Check sheet for the drawn part. Datum: minimum x, y, z corner. Units: mm. A direction names the side the tool comes from. Round coordinates to 2 decimals unless told otherwise and drop trailing zeros. Write each loop counter-clockwise with the first axis right and the second up, starting at its lowest first coordinate (ties: lowest second). Pieces come first, ordered by that corner, then holes. Notation, with made-up numbers: M -21,47.5 L 8,47.5 A13 ccw 8,59.5 Z; hole C -31,55.5 d2. An arc over 180 degrees is marked long. Answer in a Markdown table with one row per item. Add a question column.
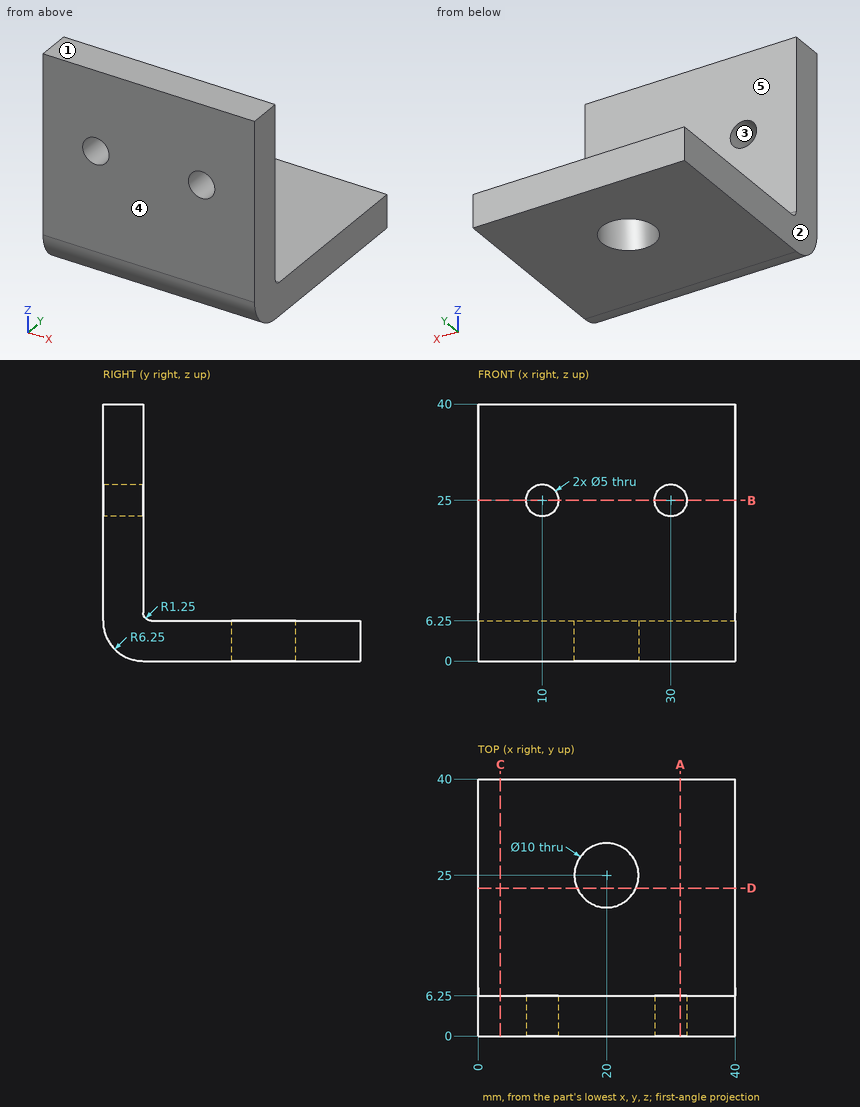
Item 1: Gauge pin test, flat end, axial feed: pin 1 Ø1 at (x, y) = (7, 25.5) entering from +Z. Record the tip position at first contact, or that the pin passes through.
Item 2: Mould release check, pull along X, two halves, no side actions. Record for the marked faces 1, 2 and 3: +X half, -X half, draft (parallel to the pull), parting line (faces both ways), or undercut.
Item 3: Section check D-D, the plane y = 23. Record the boundary of the cut face in (x, z).
Item 4: Section check C-C, the plane x = 3.5. Record the boundary of the cut face in (y, z).
Item 5: Section check A-A, the plane x = 31.5. Record the boundary of the cut face in (y, z), and give its area (3 significant figures).
Item 6: Scan lines: probe 1 along Z at (x, y) = (30, 27); probe 2 along Y at (x, z) = (20, 2.5). Record each from-to range of solid material in increasing order. Write a range as from..to.
Item 7: Access from +Z, -Z, +X, -X, +Y, -Y to the whole of each face (thin tool, end or side, straight path). Record for the marked faces 4 and 5.
Item 8: Section check B-B, the plane z = 25. Record the boundary of the cut face in (x, y), and give its area (4 significant figures).
Result sheet:
| question | item | result |
|---|---|---|
| 1 | pin 1 | stops at z = 6.25 |
| 2 | face 1 | draft |
| 2 | face 2 | -X half |
| 2 | face 3 | undercut |
| 3 | outline | M 0,0 L 15.42,0 L 15.42,6.25 L 0,6.25 Z; M 24.58,0 L 40,0 L 40,6.25 L 24.58,6.25 Z |
| 4 | outline | M 0,6.25 A6.25 ccw 6.25,0 L 40,0 L 40,6.25 L 7.5,6.25 A1.25 cw 6.25,7.5 L 6.25,40 L 0,40 Z |
| 5 | outline | M 0,6.25 A6.25 ccw 6.25,0 L 40,0 L 40,6.25 L 7.5,6.25 A1.25 cw 6.25,7.5 L 6.25,23 L 0,23 Z; M 0,27 L 6.25,27 L 6.25,40 L 0,40 Z |
| 5 | area | 428 mm^2 |
| 6 | probe 1 | z = 0..6.25 |
| 6 | probe 2 | y = 1.25..20, 30..40 |
| 7 | face 4 | +Z, -Z, +X, -X, -Y |
| 7 | face 5 | +Z, +X, -X, +Y |
| 8 | outline | M 0,0 L 7.5,0 L 7.5,6.25 L 0,6.25 Z; M 12.5,0 L 27.5,0 L 27.5,6.25 L 12.5,6.25 Z; M 32.5,0 L 40,0 L 40,6.25 L 32.5,6.25 Z |
| 8 | area | 187.5 mm^2 |
